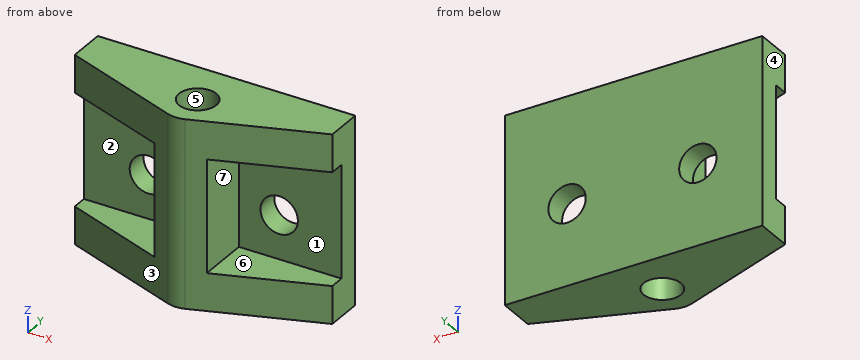
from build123d import *

# Parameters (mm, degrees)
CROQUIS2_R              = 1.5
SALIENTE_EXTRUIR2_DEPTH = 15
CROQUIS3_R              = 1.5
CORTAR_EXTRUIR1_DEPTH   = 7.633866032
CORTAR_EXTRUIR2_DEPTH   = 9
CORTAR_EXTRUIR3_DEPTH   = 9


with BuildPart() as part:
    # Croquis2 → Saliente-Extruir2 (new body)
    with BuildSketch(Plane.XY):
        with BuildLine():
            Line((-0.684040287, -2.751029697), (-10.336618829, 0.762221577))
            Line((-10.336618829, 0.762221577), (-10.336618829, 3.762221577))
            Line((-10.336618829, 3.762221577), (10.336618829, 3.762221577))
            Line((10.336618829, 3.762221577), (10.336618829, 0.762221577))
            Line((10.336618829, 0.762221577), (0.684040287, -2.751029697))
            ThreePointArc((0.684040287, -2.751029697), (0, -2.871644455), (-0.684040287, -2.751029697))
        make_face()
        Circle(CROQUIS2_R, mode=Mode.SUBTRACT)
    extrude(amount=SALIENTE_EXTRUIR2_DEPTH)

    # Croquis3 → Cortar-Extruir1 (cut, through all)
    with BuildSketch(Plane(origin=(0, 3.762221577, 0), x_dir=(1, 0, 0), z_dir=(0, 1, 0))):
        with Locations((5.336618829, -6.5)):
            Circle(CROQUIS3_R)
        with Locations((-5.163381171, -6.5)):
            Circle(CROQUIS3_R)
    extrude(amount=-CORTAR_EXTRUIR1_DEPTH, mode=Mode.SUBTRACT)

    # Croquis4 → Cortar-Extruir2 (cut)
    with BuildSketch(Plane.XY.offset(12)):
        Polygon((10.336618829, 0.762221577), (10.336618829, 1.962221577), (2.103415276, 1.962221577), (2.103415276, -2.234419449), align=None)
    extrude(amount=-CORTAR_EXTRUIR2_DEPTH, mode=Mode.SUBTRACT)

    # Croquis5 → Cortar-Extruir3 (cut)
    with BuildSketch(Plane.XY.offset(12)):
        Polygon((-10.336618829, 0.762221577), (-2.09418657, -2.237778423), (-2.09418657, 1.962221577), (-10.336618829, 1.962221577), align=None)
    extrude(amount=-CORTAR_EXTRUIR3_DEPTH, mode=Mode.SUBTRACT)


solid = part.part
CAD build for the part. Positions are in the model's coordinates, mm. Face numbers are marked on the shaded views. A direction names the side the tool comes from. Round coordinates to 2 decimals unless told otherwise and drop trailing zeros. Loops run counter-clockwise (first coordinate to the right, second up) from the corner with the lowest first, then second, coordinate; pieces in that order, holes last.
(1) Which spindle directions (+Z, -Z, +X, -X, +Y, -Y) get a long thin tool onto all of the face, cutting with end or side? Do the marked faces 1, 2 and 3. Say none if no direction does.
(2) Cut at B-B (x = 0). Give the cut face in (y, z), plus the area to 3 significant figures.
(3) Cut at C-C (z = 14.25). Give the cut face in (x, y), plus the area to 3 significant figures.
(4) Cut at A-A (z = 6.5). Give the cut face in (x, y), plus the area to 3 significant figures.
(5) Two-plate mould, pull along X, no slides. Class the marked faces 4, 5, 6 and 7: +X half, -X half, draft (parallel to the pull), parting line (faces both ways), or undercut.
(6) Wall check: line 1 along X through (y, z) = (2.45, 6.5); line 2 along Z through (x, y) = (6, 1.5); line 3 along Y through (x, z) = (0, 3). Give the ranges that are in metal, low to high.
(7) Cut at D-D (y = 0). Give the cut face in (x, z).
(8) Drop flat-ended pins along their axis: pin 1 (2.5 mm diameter, centred on x = -7.5, z = 9.5, fed in from -Y); pin 2 (1 mm diameter, centred on y = -1.5, z = 8.5, fed in from +X); pin 3 (2 mm diameter, centred on y = -1, z = 6, fed in from -X). Give the stop position or say it passes through.
Findings below:
1. face 1: +X, -Y
1. face 2: -X, -Y
1. face 3: +Z, -Z, -X, -Y
2. outline: (-2.87, 0) - (-1.5, 0) - (-1.5, 15) - (-2.87, 15) - close; (1.5, 0) - (3.76, 0) - (3.76, 15) - (1.5, 15) - close
2. area: 54.5 mm2
3. outline: (-10.34, 0.76) - (-0.68, -2.75) arc R2 ccw to (0.68, -2.75) - (10.34, 0.76) - (10.34, 3.76) - (-10.34, 3.76) - close; hole circle Ø3 at (0, 0)
3. area: 93.8 mm2
4. outline: (-10.34, 1.96) - (-6.66, 1.96) - (-6.66, 3.76) - (-10.34, 3.76) - close; (-3.66, 1.96) - (-2.09, 1.96) - (-2.09, -2.24) - (-0.68, -2.75) arc R2 ccw to (0.68, -2.75) - (2.1, -2.23) - (2.1, 1.96) - (3.84, 1.96) - (3.84, 3.76) - (-3.66, 3.76) - close; (6.84, 1.96) - (10.34, 1.96) - (10.34, 3.76) - (6.84, 3.76) - close; hole circle Ø3 at (0, 0)
4. area: 38.5 mm2
5. face 4: -X half
5. face 5: undercut
5. face 6: draft
5. face 7: +X half
6. line 1: x = -10.34 to -6.66, -3.66 to 3.84, 6.84 to 10.34
6. line 2: z = 0 to 3, 12 to 15
6. line 3: y = -2.87 to -1.5, 1.5 to 3.76
7. outline: (-8.24, 0) - (-1.5, 0) - (-1.5, 15) - (-8.24, 15) - (-8.24, 12) - (-2.09, 12) - (-2.09, 3) - (-8.24, 3) - close; (1.5, 0) - (8.24, 0) - (8.24, 3) - (2.1, 3) - (2.1, 12) - (8.24, 12) - (8.24, 15) - (1.5, 15) - close
8. pin 1: stops at y = 1.96
8. pin 2: stops at x = 2.1
8. pin 3: stops at x = -2.09
